Input: part model. Units: mm. Frame: model coordinates. Face numbers are marked on the shaded views. A direction names the side the tool comes from. Give positions to 0.01 mm unless a question says otherwise; leave off trailing zeros. Loops run counter-clockwise (first coordinate to the right, second up) from the corner with the lowest first, then second, coordinate; pieces in that order, holes last. Notation, with made-up numbers: (85, 54) - (126, 54) arc R30 ccw to (126, 82) - close; hole circle Ø4 at (-1, -36). An arc over 180 degrees is marked (long way). Answer as a JSON object with one key per item and string values.
from build123d import *

# Parameters (mm, degrees)
F0_W     = 46.99
F0_H     = 3.81
F1_DEPTH = 12.7
F3_DEPTH = 5.08


with BuildPart() as f1:
    # F0 (on Top) → F1 (new body)
    with BuildSketch(Plane.XY):
        Polygon((0, 50.8), (0, 0), (3.81, 0), (3.81, 46.99), (3.81, 50.8), align=None)
        with Locations((27.305, 48.895)):
            Rectangle(F0_W, F0_H)
    extrude(amount=F1_DEPTH)

    # F2 (on face) → F3 (join)
    with BuildSketch(Plane.XY.offset(12.7)):
        Polygon((45.72, 46.99), (3.81, 46.99), (3.81, 5.08), align=None)
        Polygon((8.6359983861, 42.1640016139), (34.0690092442, 42.1640016139), (8.6359983861, 16.7309907558), align=None, mode=Mode.SUBTRACT)
    extrude(amount=-F3_DEPTH)


solid = f1.part
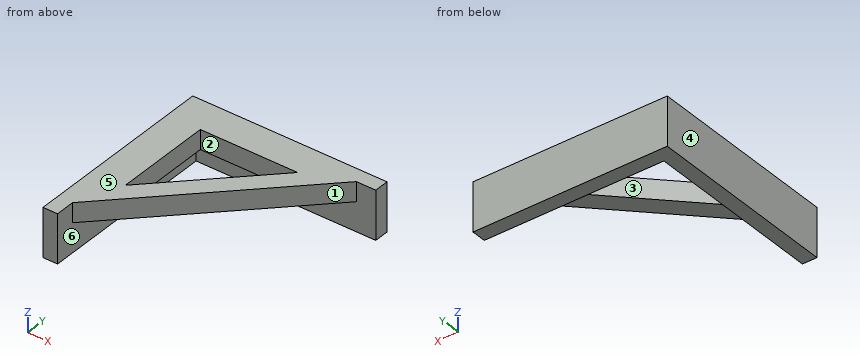
Item 1: Cut plane C-C (x = 10). Return loops of the section in (y, z) (3 decimals).
Geometry check:
{"outline": "(11.27, 7.62) - (18.095, 7.62) - (18.095, 12.7) - (11.27, 12.7) - close; (42.164, 7.62) - (46.99, 7.62) - (46.99, 0) - (50.8, 0) - (50.8, 12.7) - (42.164, 12.7) - close"}
Item 2: Material intervals for line 1 (X direction, y = 37.5, z = 2.25); line 2 (Y direction, x = 6, z = 5.25); line 3 (Z direction, x = 8.5, y = 25), sorted ascending. Write a range as [from, to].
Geometry check:
{"line 1": "x = [0, 3.81]", "line 2": "y = [46.99, 50.8]", "line 3": "z = [7.62, 12.7]"}
Item 3: Cut plane B-B (y = 29). Return loops of the section in (x, z) (3 decimals).
Geometry check:
{"outline": "(0, 0) - (3.81, 0) - (3.81, 7.62) - (8.636, 7.62) - (8.636, 12.7) - (0, 12.7) - close; (20.905, 7.62) - (27.73, 7.62) - (27.73, 12.7) - (20.905, 12.7) - close"}
Item 4: Mould query, pull axis X, two halves, no side actions, for the marked faces 1, 2, 3 and 4. Classes: released by +X, released by -X, zero draft, split by the parting line, or undercut.
Geometry check:
{"face 1": "released by +X", "face 2": "undercut", "face 3": "undercut", "face 4": "released by -X"}
Item 5: Cut plane A-A (z = 9). Return loops of the section in (x, y), then the cut area to 3 significant figures.
Geometry check:
{"outline": "(0, 0) - (3.81, 0) - (3.81, 5.08) - (45.72, 46.99) - (50.8, 46.99) - (50.8, 50.8) - (0, 50.8) - close; hole (8.64, 16.73) - (34.07, 42.16) - (8.64, 42.16) - close", "area": "927 mm2"}
Item 6: Cut plane D-D (y = 8). Return loops of the section in (x, z).
Geometry check:
{"outline": "(0, 0) - (3.81, 0) - (3.81, 7.62) - (6.73, 7.62) - (6.73, 12.7) - (0, 12.7) - close"}
Item 7: Access query for the marked faces 5 and 6. Directions: +Z, -Z, +X, -X, +Y, -Y. A direction counts if a zero-diameter tool reaches every point of the face in a straight line with its end or side. Return the directions, or none.
Geometry check:
{"face 5": "+Z, +X, -X, +Y, -Y", "face 6": "-Z, +X, -Y"}
Item 8: Contact query for flat-ended pins moving along their axis: P1, Ø12, axis at x = 24.5, y = 37.5, coming from the +Z side; P2, Ø1.5, axis at x = 17, z = 11, coming from the -Y side; P3, Ø1.5, axis at y = 21, z = 2.5, coming from the +X side; P4, Ø12.5, axis at x = 15, y = 36, coming from the -Z side. Output: stop coordinate, or through.
Geometry check:
{"P1": "stops at z = 12.7", "P2": "stops at y = 17.52", "P3": "stops at x = 3.81", "P4": "stops at z = 7.62"}
